```python
from build123d import *

# Parameters (mm, degrees)
BOSS_EXTRUDE3_DEPTH = 12
SKETCH5_W           = 3
SKETCH5_H           = 18
BOSS_EXTRUDE4_DEPTH = 4.5
CHAMFER1_SIZE       = 1
SKETCH4_R           = 1.85
CUT_EXTRUDE1_DEPTH  = 12


with BuildPart() as part:
    # Sketch3 → Boss-Extrude3 (new body)
    with BuildSketch(Plane.ZY.offset(178.52034041)):
        Polygon((-3, 14.684603209), (-5.250229512, 12.884419599), (-3, 11.084235989), (-3, 8.134419599), (0, 8.134419599), (0, 17.634419599), (-3, 17.634419599), align=None)
    extrude(amount=-BOSS_EXTRUDE3_DEPTH)

    # Sketch5 → Boss-Extrude4 (add, symmetric)
    with BuildSketch(Plane(origin=(-166.52034041, 0, 0), x_dir=(0, 0, -1), z_dir=(1, 0, 0))):
        with Locations((1.5, 17.134419599)):
            Rectangle(SKETCH5_W, SKETCH5_H)
    extrude(amount=BOSS_EXTRUDE4_DEPTH, both=True)

    # Chamfer1
    chamfer1_edges = [part.edges().sort_by_distance(p)[0] for p in [
        (-171.02034041, 17.634419599, -1.5),
        (-171.02034041, 26.134419599, -1.5),
        (-162.02034041, 8.134419599, -1.5),
        (-162.02034041, 26.134419599, -1.5),
        (-178.52034041, 17.634419599, -1.5),
        (-178.52034041, 8.134419599, -1.5),
    ]]
    chamfer(chamfer1_edges, length=CHAMFER1_SIZE)

    # Sketch4 → Cut-Extrude1 (cut)
    with BuildSketch(Plane.XY):
        with Locations((-172.52034041, 13.134419599)):
            Circle(SKETCH4_R)
    extrude(amount=-CUT_EXTRUDE1_DEPTH, mode=Mode.SUBTRACT)


solid = part.part
```
Work out the finished part from the listing and answer in its coordinate system (mm). A direction names the side the tool comes from. Coordinates: 2 decimals unless noted, no trailing zeros. Loops run counter-clockwise (first coordinate to the right, second up) from the corner with the lowest first, then second, coordinate; pieces in that order, holes last. Notation, with made-up numbers: (77.5, -31.5) -> (90.5, -31.5) arc R25 ccw to (90.5, -6.5) -> close; hole circle Ø10 at (-32, 67.5). An arc over 180 degrees is marked (long way). Answer as CSV lines item,"result".
Q1. A tool of negligible diameter and unlimited length cuts with its end or side. For faces 4 (the face through (-170, 8.134, -1)), 5 (the face through (-175, 17.634, -1)), from which of +Z, -Z, +X, -X, +Y, -Y can it reach the whole face along a straight path? Write none if from no direction.
Findings:
face 4,"+Z, -Z, +X, -X, -Y"
face 5,"+Z, -Z, -X, +Y"
Q2. The part is cut by section B-B on y = 13.75. Write down the section's boundary in (x, z), and give its area (3 significant figures).
Findings:
outline,"(-178.52, -4.17) -> (-174.26, -4.17) -> (-174.26, 0) -> (-178.52, 0) -> close; (-170.78, -4.17) -> (-166.52, -4.17) -> (-166.52, -3) -> (-162.02, -3) -> (-162.02, 0) -> (-170.78, 0) -> close"
area,"49.0 mm²"
Q3. The part is cut by section A-A on x = -176.5. Write down the section's boundary in (y, z), and give its area (3 significant figures).
Findings:
outline,"(8.13, -3) -> (11.08, -3) -> (12.88, -5.25) -> (14.68, -3) -> (17.63, -3) -> (17.63, 0) -> (8.13, 0) -> close"
area,"32.6 mm²"
Q4. Each of these flat-tipped pins is pushed along its axis until it touches: pin 1 (1 mm diameter, centred on x = -170, y = 22, fed in from -Z); pin 2 (1.5 mm diameter, centred on x = -176, z = -1.5, fed in from +Y); pin 3 (0.9 mm diameter, centred on y = 22, z = -1, fed in from -X). Where does it stop, or does it pass through?
Findings:
pin 1,"stops at z = -3"
pin 2,"stops at y = 17.63"
pin 3,"stops at x = -171.02"
Q5. The part is cut by section C-C on z = -3.65. Write down the section's boundary in (x, y), and give its area (3 significant figures).
Findings:
outline,"(-178.52, 11.6) -> (-173.56, 11.6) arc R1.85 cw to (-174.06, 14.16) -> (-178.52, 14.16) -> close; (-171.48, 11.6) -> (-166.52, 11.6) -> (-166.52, 14.16) -> (-170.98, 14.16) arc R1.85 cw to start"
area,"22.2 mm²"
Q6. The part is cut by section D-D on x = -172.75. Write down the section's boundary in (y, z).
Findings:
outline,"(8.13, -3) -> (11.08, -3) -> (11.3, -3.27) -> (11.3, 0) -> (8.13, 0) -> close; (14.97, -3) -> (17.63, -3) -> (17.63, 0) -> (14.97, 0) -> close"
Q7. Find the intervals of material crossed by probe 1 along X at (y, z) = (13.25, -0.6); probe 2 along Z at (x, y) = (-168.25, 25.25); probe 3 along X at (y, z) = (21.75, -1.1), in increasing order.
Findings:
probe 1,"x = -178.52 to -174.37, -170.67 to -162.02"
probe 2,"z = -3 to 0"
probe 3,"x = -171.02 to -162.02"
Q8. For a pull along X with two mould halves and no side action, classify faces 1 (the face through (-171.02, 22, -1)), 2 (the face through (-172.92, 11.33, -2.01)), 3 (the face through (-166.52, 13, -4)) as +X half, -X half, draft (parallel to the pull), parting line (faces both ways), or undercut.
Findings:
face 1,"-X half"
face 2,"undercut"
face 3,"+X half"
